```python
from build123d import *

# Parameters (mm, degrees)
SKETCH1_W           = 142
SKETCH1_H           = 92
BOSS_EXTRUDE1_DEPTH = 14
FILLET1_R           = 10
SKETCH2_R           = 27.5
SKETCH2_R_2         = 15
BOSS_EXTRUDE2_DEPTH = 22.5
BOSS_EXTRUDE3_DEPTH = 7.5
RIB1_START          = -7.5
RIB1_DEPTH          = 15
SKETCH6_R           = 6.879028827
CUT_EXTRUDE1_DEPTH  = 121.279881942


with BuildPart() as part:
    # Sketch1 → Boss-Extrude1 (new body)
    with BuildSketch(Plane(origin=(0, 0, 0), x_dir=(1, 0, 0), z_dir=(0, 1, 0))):
        Rectangle(SKETCH1_W, SKETCH1_H)
    extrude(amount=BOSS_EXTRUDE1_DEPTH)

    # Fillet1
    fillet1_edges = [part.edges().sort_by_distance(p)[0] for p in [
        (71, 7, 46),
        (-71, 7, 46),
        (-71, 7, -46),
        (71, 7, -46),
    ]]
    fillet(fillet1_edges, radius=FILLET1_R)



with BuildPart() as body_2:
    # Sketch2 → Boss-Extrude2 (new, symmetric)
    with BuildSketch(Plane(origin=(0, 0, 0), x_dir=(0, 0, -1), z_dir=(1, 0, 0))):
        with Locations(Location((0, 72, 0), (0, 0, 180))):
            Circle(SKETCH2_R)
        with Locations(Location((0, 72, 0), (0, 0, 180))):
            Circle(SKETCH2_R_2, mode=Mode.SUBTRACT)
    extrude(amount=BOSS_EXTRUDE2_DEPTH, both=True)


with BuildPart() as part_1:
    add(part.part)

    add(body_2.part)  # Boss-Extrude3 merges body 2
    # Sketch4 → Boss-Extrude3 (add, symmetric)
    with BuildSketch(Plane(origin=(0, 0, 0), x_dir=(0, 0, -1), z_dir=(1, 0, 0))):
        with BuildLine():
            Line((-25.148338126, 83.127043161), (-46, 36))
            Line((-46, 36), (-46, 14))
            Line((-46, 14), (46, 14))
            Line((46, 14), (46, 36))
            Line((46, 36), (25.148338126, 83.127043161))
            ThreePointArc((25.148338126, 83.127043161), (0, 44.5), (-25.148338126, 83.127043161))
        make_face()
    extrude(amount=BOSS_EXTRUDE3_DEPTH, both=True)

    # Rib1: read off the stored shape, not the designer's step
    # Rib1 outline → Rib1 (add)
    with BuildSketch(Plane.XY.offset(RIB1_START)):
        Polygon((-7.5, 14), (-7.5, 45.542486889), (-22.5, 45.542486889), (-22.5, 44.5), (-71, 14), align=None)
    rib1 = extrude(amount=RIB1_DEPTH)

    # Mirror1: Rib1 across plane
    add(rib1.mirror(Plane(origin=(0, 0, 0), x_dir=(0, 0, 1), z_dir=(1, 0, 0))))

    # Sketch6 → Cut-Extrude1 (cut, through all)
    with BuildSketch(Plane(origin=(0, 14, 0), x_dir=(1, 0, 0), z_dir=(0, 1, 0))):
        with Locations(Location((-48.5, 25, 0), (0, 0, 270))):
            Circle(SKETCH6_R)
        with Locations(Location((-48.5, -25, 0), (0, 0, 270))):
            Circle(SKETCH6_R)
        with Locations(Location((48.5, 25, 0), (0, 0, 270))):
            Circle(SKETCH6_R)
        with Locations(Location((50.121402644, -25, 0), (0, 0, 270))):
            Circle(SKETCH6_R)
    extrude(amount=-CUT_EXTRUDE1_DEPTH, mode=Mode.SUBTRACT)


solid = part_1.part
```
Read the model definition and answer for the solid it produces. Units are mm, in the model's axes. A direction names the side the tool comes from. Give positions to 0.01 mm unless a question says otherwise; leave off trailing zeros. Write each loop counter-clockwise with the first axis right and the second up, starting at its lowest first coordinate (ties: lowest second). Pieces come first, ordered by that corner, then holes. Notation, with made-up numbers: M 64.5,36 L 123.5,36 A19 cw 123.5,66 Z; hole C 79,24.5 d10. An arc over 180 degrees is marked long. Put each result on its own line as item: value. Start each with the question number.
1. Each of these flat-tipped pins is pushed along its axis until it touches: pin 1 Ø16.5 at (y, z) = (84.5, 3.5) entering from +X; pin 2 Ø5 at (y, z) = (38.5, -5) entering from +X; pin 3 Ø9.5 at (x, y) = (33.5, 23.5) entering from -Z. Where does it stop, or does it pass through?
2. The part is cut by section B-B, the plane x = 48.5. Give the vertices of the cut face in (y, z), and give its area (3 significant figures).
3. Consider line 1 along X through (y, z) = (3, 25); line 2 along X through (y, z) = (9.5, -25); line 3 along Y through (x, z) = (-64, 8.5). Determine where each line is inside the solid, lowest interval first.
4. Which of the six approach directions +Z, -Z, +X, -X, +Y, -Y give full straight-line access (tool end or side, diameter ignored) to faces 4 (the flat face through (-7.5, 34, -26)), 5 (the flat face through (-40, 14, 26)), 6 (the flat face through (39, 14, 26))?
5. The part is cut by section D-D, the plane z = 21. Give the vertices of the cut face in (x, y).
6. The part is cut by section C-C, the plane y = 72. Give the vertices of the cut face in (x, z).
7. The part is cut by section A-A, the plane z = 0. Give the vertices of the cut face in (x, y).
8. For a pull along Y with two mould halves and no side action, classify faces 1 (the flat face through (7.5, 34, -26)), 2 (the flat face through (-46.41, 29.464, -0.105)), 3 (the cylindrical face through (-46.43, 7.1, 31.56)) as released by +Y, released by -Y, zero draft, split by the parting line, or undercut.
Final values:
1. pin 1: stops at x = 22.5
1. pin 2: stops at x = 36.02
1. pin 3: stops at z = -7.5
2. outline: M 0,-46 L 14,-46 L 14,-31.88 L 0,-31.88 Z; M 0,-18.12 L 14,-18.12 L 14,-7.5 L 28.15,-7.5 L 28.15,7.5 L 14,7.5 L 14,18.31 L 0,18.31 Z; M 0,31.69 L 14,31.69 L 14,46 L 0,46 Z
2. area: 1,120 mm²
3. line 1: x = -71 to -55.38, -41.62 to 43.24, 57 to 71
3. line 2: x = -71 to -55.38, -41.62 to 41.62, 55.38 to 71
3. line 3: y = 0 to 14
4. face 4: -Z, -X
4. face 5: +Z, -X
4. face 6: +Z, +X
5. outline: M -71,0 L -54.1,0 L -54.1,14 L -71,14 Z; M -42.9,0 L 44.52,0 L 44.52,14 L 7.5,14 L 7.5,54.24 L 22.5,54.24 L 22.5,89.76 L -22.5,89.76 L -22.5,54.24 L -7.5,54.24 L -7.5,14 L -42.9,14 Z; M 55.72,0 L 71,0 L 71,14 L 55.72,14 Z
6. outline: M -22.5,-27.5 L -7.5,-27.5 L -7.5,-30.07 L 7.5,-30.07 L 7.5,-27.5 L 22.5,-27.5 L 22.5,-15 L -22.5,-15 Z; M -22.5,15 L 22.5,15 L 22.5,27.5 L 7.5,27.5 L 7.5,30.07 L -7.5,30.07 L -7.5,27.5 L -22.5,27.5 Z
7. outline: M -71,0 L 71,0 L 71,14 L 22.5,44.5 L 22.5,57 L -22.5,57 L -22.5,44.5 L -71,14 Z; M -22.5,87 L 22.5,87 L 22.5,99.5 L -22.5,99.5 Z
8. face 1: undercut
8. face 2: released by +Y
8. face 3: zero draft
